```python
from build123d import *

# Parameters (mm, degrees)
SKETCH2_W           = 25.4
SKETCH2_H           = 25.4
BOSS_EXTRUDE1_DEPTH = 279.4
SKETCH4_W           = 19.05
SKETCH4_H           = 19.05
CUT_EXTRUDE1_DEPTH  = 280.9766776
SKETCH5_R           = 3.2639
CUT_EXTRUDE2_DEPTH  = 281.839473721
SKETCH6_R           = 3.2639
CUT_EXTRUDE3_DEPTH  = 281.839473721
SKETCH7_R           = 3.2639
CUT_EXTRUDE4_DEPTH  = 281.839473721


with BuildPart() as part:
    # Sketch2 → Boss-Extrude1 (new body)
    with BuildSketch(Plane.XY):
        Rectangle(SKETCH2_W, SKETCH2_H)
    extrude(amount=BOSS_EXTRUDE1_DEPTH)

    # Sketch4 → Cut-Extrude1 (cut, through all)
    with BuildSketch(Plane.XY):
        Rectangle(SKETCH4_W, SKETCH4_H)
    extrude(amount=CUT_EXTRUDE1_DEPTH, mode=Mode.SUBTRACT)

    # Sketch5 → Cut-Extrude2 (cut, through all)
    with BuildSketch(Plane(origin=(0, 12.7, 0), x_dir=(1, 0, 0), z_dir=(0, 1, 0))):
        with Locations(Location((0, -15.24, 0), (0, 0, 270))):
            Circle(SKETCH5_R)
    extrude(amount=-CUT_EXTRUDE2_DEPTH, mode=Mode.SUBTRACT)

    # Sketch6 → Cut-Extrude3 (cut, through all)
    with BuildSketch(Plane(origin=(0, 12.7, 0), x_dir=(1, 0, 0), z_dir=(0, 1, 0))):
        with Locations(Location((0, -228.6, 0), (0, 0, 270))):
            Circle(SKETCH6_R)
    extrude(amount=-CUT_EXTRUDE3_DEPTH, mode=Mode.SUBTRACT)

    # Sketch7 → Cut-Extrude4 (cut, through all)
    with BuildSketch(Plane.ZY.offset(12.7)):
        with Locations((15.24, 0)):
            Circle(SKETCH7_R)
    extrude(amount=-CUT_EXTRUDE4_DEPTH, mode=Mode.SUBTRACT)


solid = part.part
```
Check sheet for the modelled part. Datum: model origin and axes. Units: mm. A direction names the side the tool comes from. Round coordinates to 2 decimals unless told otherwise and drop trailing zeros. Write each loop counter-clockwise with the first axis right and the second up, starting at its lowest first coordinate (ties: lowest second). Pieces come first, ordered by that corner, then holes. Notation, with made-up numbers: (-32.5, 16.25) -> (2.5, 16.25) arc R18 ccw to (2.5, 44.25) -> close; hole circle Ø2 at (75.5, 72.25). An arc over 180 degrees is marked (long way). Put each result on its own line as item: value.
(1) Sectioned sample at B-B (y = 0). Enter the section's corners in (x, z) (3 decimals).
Values found:
outline: (-12.7, 0) -> (-9.525, 0) -> (-9.525, 11.976) -> (-12.7, 11.976) -> close; (-12.7, 18.504) -> (-9.525, 18.504) -> (-9.525, 279.4) -> (-12.7, 279.4) -> close; (9.525, 0) -> (12.7, 0) -> (12.7, 11.976) -> (9.525, 11.976) -> close; (9.525, 18.504) -> (12.7, 18.504) -> (12.7, 279.4) -> (9.525, 279.4) -> close
(2) Sectioned sample at D-D (z = 15.24). Enter the section's corners in (x, y) (3 decimals).
Values found:
outline: (-12.7, -12.7) -> (-3.264, -12.7) -> (-3.264, -9.525) -> (-9.525, -9.525) -> (-9.525, -3.264) -> (-12.7, -3.264) -> close; (-12.7, 3.264) -> (-9.525, 3.264) -> (-9.525, 9.525) -> (-3.264, 9.525) -> (-3.264, 12.7) -> (-12.7, 12.7) -> close; (3.264, -12.7) -> (12.7, -12.7) -> (12.7, -3.264) -> (9.525, -3.264) -> (9.525, -9.525) -> (3.264, -9.525) -> close; (3.264, 9.525) -> (9.525, 9.525) -> (9.525, 3.264) -> (12.7, 3.264) -> (12.7, 12.7) -> (3.264, 12.7) -> close
(3) Sectioned sample at A-A (z = 228.6). Enter the section's corners in (x, y) (3 decimals).
Values found:
outline: (-12.7, -12.7) -> (-3.264, -12.7) -> (-3.264, -9.525) -> (-9.525, -9.525) -> (-9.525, 9.525) -> (-3.264, 9.525) -> (-3.264, 12.7) -> (-12.7, 12.7) -> close; (3.264, -12.7) -> (12.7, -12.7) -> (12.7, 12.7) -> (3.264, 12.7) -> (3.264, 9.525) -> (9.525, 9.525) -> (9.525, -9.525) -> (3.264, -9.525) -> close
(4) Sectioned sample at C-C (x = 0). Enter the section's corners in (y, z) (3 decimals).
Values found:
outline: (-12.7, 0) -> (-9.525, 0) -> (-9.525, 11.976) -> (-12.7, 11.976) -> close; (-12.7, 18.504) -> (-9.525, 18.504) -> (-9.525, 225.336) -> (-12.7, 225.336) -> close; (-12.7, 231.864) -> (-9.525, 231.864) -> (-9.525, 279.4) -> (-12.7, 279.4) -> close; (9.525, 0) -> (12.7, 0) -> (12.7, 11.976) -> (9.525, 11.976) -> close; (9.525, 18.504) -> (12.7, 18.504) -> (12.7, 225.336) -> (9.525, 225.336) -> close; (9.525, 231.864) -> (12.7, 231.864) -> (12.7, 279.4) -> (9.525, 279.4) -> close
(5) Tool access check on faces 4 (the face through (11.09, -1.25, 18.255)), 5 (the face through (0, 9.525, 138)). Record the directions out of +Z, -Z, +X, -X, +Y, -Y that give a thin tool (end or side, any length) a straight path to the whole face; none if there is none.
Values found:
face 4: +X, -X
face 5: +Z, -Z
(6) Material ranges on line 1 (X direction, y = -8.25, z = 103.5) (3 decimals); line 2 (Y direction, x = -11.9, z = 15.24), recorded low to high.
Values found:
line 1: x = -12.7 to -9.525, 9.525 to 12.7
line 2: y = -12.7 to -3.26, 3.26 to 12.7
(7) Mould release check, pull along Y, two halves, no side actions. Record for faces 1 (the face through (0, -12.7, 138)), 2 (the face through (-9.525, 0, 138)), 3 (the face through (-1.25, -11.09, 18.255)): released by +Y, released by -Y, zero draft, split by the parting line, or undercut.
Values found:
face 1: released by -Y
face 2: undercut
face 3: zero draft
